Verification items for this drawing (mm, ordinates from the low corner). Round coordinates to 2 decimals unless told otherwise and drop trailing zeros. Order: outer loops, then holes, each group sorted by start corner. A loop starts at its lowest first (then second) coordinate and runs counter-clockwise, first axis right, second up. Notation, with made-up numbers: (44.25, 0) - (103.25, 0) arc R11 cw to (103.25, 10) - close; hole circle Ø10 at (52.25, -16). An arc over 180 degrees is marked (long way). Use a Markdown table: item, result. Add a question column.
(1) Section check C-C on y = 16.5. Record the boundary of the cut face in (x, z) (1 decimal).
(2) Thickness scan on line 1 along X through (y, z) = (21, 1.95) (1 decimal); line 2 along Y through (x, z) = (15, 1.85); line 3 along X through (y, z) = (24.5, 0.35). Record the ranges inside material, lowest first. Write a range as [from, to].
(3) Gauge pin test, flat end, axial feed: P1, Ø1, axis at y = 40, z = 1, coming from the +X side. Record the tip position at first contact, or that the pin passes through.
(4) Section check A-A on x = 56.5. Record the boundary of the cut face in (y, z).
(5) Section check D-D on y = 25. Record the boundary of the cut face in (x, z), then the cut area to 3 significant figures.
(6) Section check B-B on z = 2.1. Record the boundary of the cut face in (x, y) (1 decimal), then the cut area to 3 significant figures.
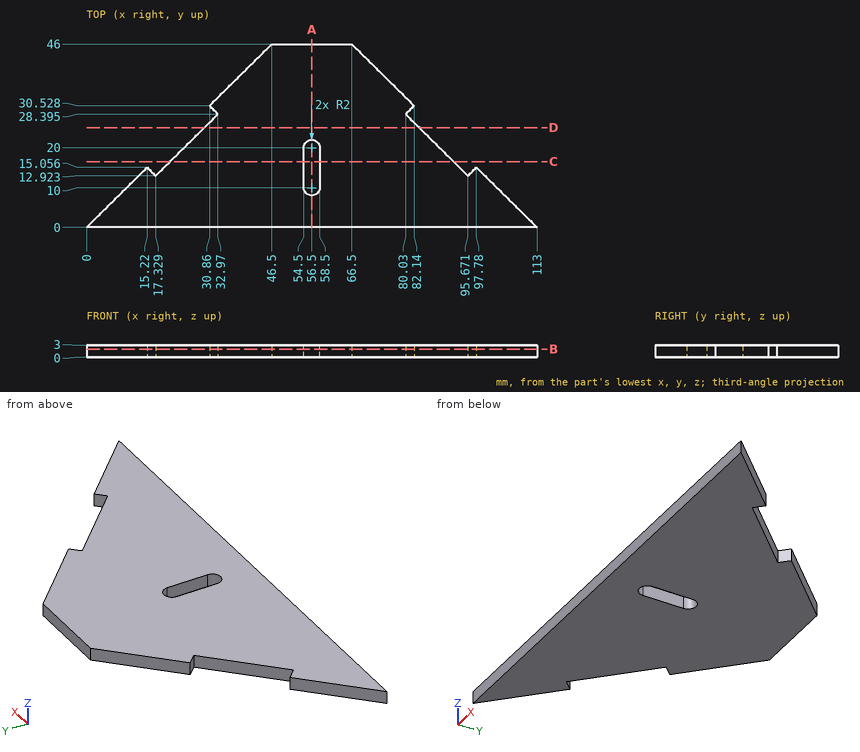
Check sheet entries:
| question | item | result |
|---|---|---|
| 1 | outline | (20.9, 0) - (54.5, 0) - (54.5, 3) - (20.9, 3) - close; (58.5, 0) - (92.1, 0) - (92.1, 3) - (58.5, 3) - close |
| 2 | line 1 | x = [25.5, 54.8], [58.2, 87.5] |
| 2 | line 2 | y = [0, 14.84] |
| 2 | line 3 | x = [29.03, 83.97] |
| 3 | P1 | stops at x = 73.07 |
| 4 | outline | (0, 0) - (8, 0) - (8, 3) - (0, 3) - close; (22, 0) - (46, 0) - (46, 3) - (22, 3) - close |
| 5 | outline | (29.54, 0) - (83.46, 0) - (83.46, 3) - (29.54, 3) - close |
| 5 | area | 162 mm2 |
| 6 | outline | (0, 0) - (113, 0) - (97.8, 15.1) - (95.7, 12.9) - (80, 28.4) - (82.1, 30.5) - (66.5, 46) - (46.5, 46) - (30.9, 30.5) - (33, 28.4) - (17.3, 12.9) - (15.2, 15.1) - close; hole (54.5, 10) arc R2 ccw to (58.5, 10) - (58.5, 20) arc R2 ccw to (54.5, 20) - close |
| 6 | area | 2,870 mm2 |
